Part model, mm, in its own coordinate system. Face numbers are marked on the shaded views. Give positions to 0.01 mm unless a question says otherwise; leave off trailing zeros. Order: outer loops, then holes, each group sorted by start corner. A loop starts at its lowest first (then second) coordinate and runs counter-clockwise, first axis right, second up.
1. Slice it at C-C on y = 10. List the corners of the cut face in (x, z), and give its area (3 significant figures).
2. Drop flat-ended pins along their axis: pin 1 Ø5 at (x, z) = (11, 8) entering from -Y; pin 2 Ø5 at (y, z) = (5, 51) entering from +X; pin 3 Ø12 at (y, z) = (10.5, 20) entering from -X. Give the stop position or say it passes through.
3. Mould opens along Z. For the marked faces 1, 2, 3 and 4 say: +Z half, -Z half, draft (parallel to the pull), parting line (faces both ways), or undercut.
4. Probe line 1 (Z direction, x = 12.5, y = 1); line 2 (X direction, y = 10.25, z = 22.5); line 3 (X direction, y = 9.25, z = 10.5). List the from-to ranges inside material, lowest first.
5. Slice it at A-A on y = 14.5. List the corners of the cut face in (x, z), and give its area (3 significant figures).
from build123d import *

# Parameters (mm, degrees)
SKETCH1_W           = 20
SKETCH1_H           = 20
BOSS_EXTRUDE1_DEPTH = 10
SKETCH4_W           = 20
SKETCH4_H           = 10
BOSS_EXTRUDE2_DEPTH = 20
FILLET6_R           = 1
FILLET7_R           = 1
SKETCH6_R           = 1
BOSS_EXTRUDE3_DEPTH = 60


with BuildPart() as part:
    # Sketch1 → Boss-Extrude1 (new body)
    with BuildSketch(Plane.XY):
        with Locations((10, 10)):
            Rectangle(SKETCH1_W, SKETCH1_H)
    extrude(amount=BOSS_EXTRUDE1_DEPTH)

    # Fillet6
    fillet6_edges = [part.edges().sort_by_distance(p)[0] for p in [
        (20, 10, 10),
        (10, 20, 10),
        (0, 10, 10),
        (10, 20, 0),
        (20, 10, 0),
        (10, 0, 0),
        (0, 10, 0),
        (0, 20, 5),
        (20, 20, 5),
        (20, 0, 5),
        (0, 0, 5),
        (10, 0, 10),
    ]]
    fillet(fillet6_edges, radius=FILLET6_R)



with BuildPart() as body_2:
    # Sketch4 → Boss-Extrude2 (new body)
    with BuildSketch(Plane(origin=(0, 0, 0), x_dir=(1, 0, 0), z_dir=(0, 1, 0))):
        with Locations((10, -65)):
            Rectangle(SKETCH4_W, SKETCH4_H)
    extrude(amount=BOSS_EXTRUDE2_DEPTH)

    # Fillet7
    fillet7_edges = [body_2.edges().sort_by_distance(p)[0] for p in [
        (20, 20, 65),
        (10, 20, 60),
        (0, 20, 65),
        (10, 0, 60),
        (20, 0, 65),
        (10, 0, 70),
        (0, 0, 65),
        (0, 10, 60),
        (20, 10, 60),
        (20, 10, 70),
        (0, 10, 70),
        (10, 20, 70),
    ]]
    fillet(fillet7_edges, radius=FILLET7_R)


with BuildPart() as part_1:
    add(part.part)

    add(body_2.part)  # Boss-Extrude3 merges body 2
    # Sketch6 → Boss-Extrude3 (add)
    with BuildSketch(Plane.XY.offset(10)):
        with Locations((10, 10)):
            Circle(SKETCH6_R)
    extrude(amount=BOSS_EXTRUDE3_DEPTH)


solid = part_1.part
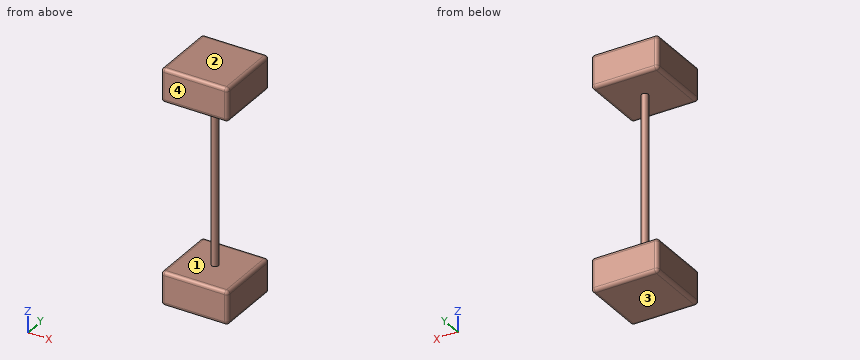
Data:
1. outline: (0, 1) arc R1 ccw to (1, 0) - (19, 0) arc R1 ccw to (20, 1) - (20, 9) arc R1 ccw to (19, 10) - (11, 10) - (11, 60) - (19, 60) arc R1 ccw to (20, 61) - (20, 69) arc R1 ccw to (19, 70) - (1, 70) arc R1 ccw to (0, 69) - (0, 61) arc R1 ccw to (1, 60) - (9, 60) - (9, 10) - (1, 10) arc R1 ccw to (0, 9) - close
1. area: 498 mm2
2. pin 1: stops at y = 0
2. pin 2: passes through
2. pin 3: stops at x = 9
3. face 1: undercut
3. face 2: +Z half
3. face 3: -Z half
3. face 4: draft
4. line 1: z = 0 to 10, 60 to 70
4. line 2: x = 9.03 to 10.97
4. line 3: x = 9.34 to 10.66
5. outline: (0, 1) arc R1 ccw to (1, 0) - (19, 0) arc R1 ccw to (20, 1) - (20, 9) arc R1 ccw to (19, 10) - (1, 10) arc R1 ccw to (0, 9) - close; (0, 61) arc R1 ccw to (1, 60) - (19, 60) arc R1 ccw to (20, 61) - (20, 69) arc R1 ccw to (19, 70) - (1, 70) arc R1 ccw to (0, 69) - close
5. area: 398 mm2
